Could you check a few things on this model? Use its own coordinates, in mm. Face numbers are marked on the shaded views. A direction names the side the tool comes from. Give positions to 0.01 mm unless a question says otherwise; leave off trailing zeros. Write each loop counter-clockwise with the first axis right and the second up, starting at its lowest first coordinate (ties: lowest second). Pieces come first, ordered by that corner, then holes. Notation, with made-up numbers: (30.5, 51) -> (53.5, 51) arc R28 ccw to (53.5, 86) -> close; hole circle Ø2 at (12.25, 12.25). An arc over 180 degrees is marked (long way). One line per question, with ' | ' between items.
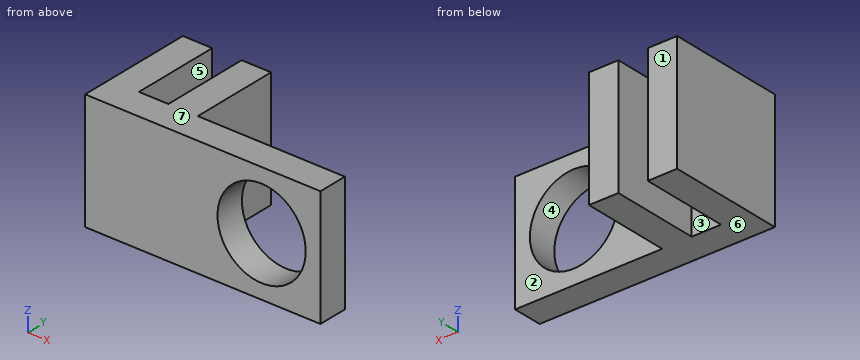
from build123d import *

# Parameters (mm, degrees)
SKETCH1_W             = 10
SKETCH1_H             = 40
BOSS_EXTRUDE1_DEPTH   = 40
BOSS_EXTRUDE1_2_DEPTH = 40
SKETCH1_3_W           = 10
SKETCH1_3_H           = 40
SKETCH1_3_W_2         = 50
SKETCH1_3_R           = 15
BOSS_EXTRUDE2_DEPTH   = 10


with BuildPart() as part:
    # Sketch1 → Boss-Extrude1 (new body)
    with BuildSketch(Plane(origin=(0, 0, 0), x_dir=(1, 0, 0), z_dir=(0, 1, 0))):
        with Locations((5, 20)):
            Rectangle(SKETCH1_W, SKETCH1_H)
    extrude(amount=BOSS_EXTRUDE1_DEPTH)



with BuildPart() as body_2:
    # Sketch1 → Boss-Extrude1 2 (new body)
    with BuildSketch(Plane(origin=(0, 0, 0), x_dir=(1, 0, 0), z_dir=(0, 1, 0))):
        with Locations((25, 20)):
            Rectangle(SKETCH1_W, SKETCH1_H)
    extrude(amount=BOSS_EXTRUDE1_2_DEPTH)


with BuildPart() as part_1:
    add(part.part)

    add(body_2.part)  # Boss-Extrude2 merges body 2
    # Sketch1_3 → Boss-Extrude2 (add)
    # profile 1 of 2: a face of its own
    with BuildSketch(Plane(origin=(0, 0, 0), x_dir=(1, 0, 0), z_dir=(0, 1, 0))):
        with Locations((15, 20)):
            Rectangle(SKETCH1_3_W, SKETCH1_3_H)
    # profile 2 of 2: a face of its own
    with BuildSketch(Plane(origin=(0, 0, 0), x_dir=(1, 0, 0), z_dir=(0, 1, 0))):
        with Locations((55, 20)):
            Rectangle(SKETCH1_3_W_2, SKETCH1_3_H)
        with Locations(Location((60, 20, 0), (0, 0, 270))):
            Circle(SKETCH1_3_R, mode=Mode.SUBTRACT)
    extrude(amount=BOSS_EXTRUDE2_DEPTH)


solid = part_1.part
Q1. On a 3-axis mill with a long thin cutter (end or side, diameter ignored), from which of +Z, -Z, +X, -X, +Y, -Y can I reach the whole of each face in a straight line? I mean the marked faces 1, 2 and 3. Say none if no direction works.
Answer below:
face 1: +Z, -Z, +X, -X, +Y | face 2: +Z, -Z, +X, +Y | face 3: +Z, -Z, +Y
Q2. If we mould it in two halves opening along Z, with no side actions, what happens to the marked faces 4, 5, 6 and 7? For each: +Z half, -Z half, draft (parallel to the pull), parting line (faces both ways), or undercut.
Answer below:
face 4: undercut | face 5: draft | face 6: -Z half | face 7: +Z half
Q3. Imagine slicing it at B-B on x = 60. Please give me the cut outline in (y, z).
Answer below:
outline: (0, -40) -> (10, -40) -> (10, -35) -> (0, -35) -> close; (0, -5) -> (10, -5) -> (10, 0) -> (0, 0) -> close
Q4. If I drill on line 1 along X through (y, z) = (6.75, -20); line 2 along X through (y, z) = (13, -26); line 3 along Y through (x, z) = (34.5, -30), over which ranges is the centre line in solid material (lowest first)?
Answer below:
line 1: x = 0 to 45, 75 to 80 | line 2: x = 0 to 10, 20 to 30 | line 3: y = 0 to 10
Q5. Will these pins go through, and if not, where does the flat tip stop? pin 1 (20 mm diameter, centred on x = 52, z = -12, fed in from +Y); pin 2 (24 mm diameter, centred on y = 31.5, z = -28.5, fed in from +X).
Answer below:
pin 1: stops at y = 10 | pin 2: stops at x = 30
Q6. Imagine slicing it at D-D on y = 9. Please give me the cut outline in (x, z), and give its area (3 significant figures).
Answer below:
outline: (0, -40) -> (80, -40) -> (80, 0) -> (0, 0) -> close; hole circle Ø30 at (60, -20) | area: 2,490 mm^2
Q7. Imagine slicing it at C-C on y = 26. Please give me the cut outline in (x, z), and give its area (3 significant figures).
Answer below:
outline: (0, -40) -> (10, -40) -> (10, 0) -> (0, 0) -> close; (20, -40) -> (30, -40) -> (30, 0) -> (20, 0) -> close | area: 800 mm^2
Q8. Imagine slicing it at A-A on z = -20. Please give me the cut outline in (x, y), and give its area (3 significant figures).
Answer below:
outline: (0, 0) -> (45, 0) -> (45, 10) -> (30, 10) -> (30, 40) -> (20, 40) -> (20, 10) -> (10, 10) -> (10, 40) -> (0, 40) -> close; (75, 0) -> (80, 0) -> (80, 10) -> (75, 10) -> close | area: 1,100 mm^2
